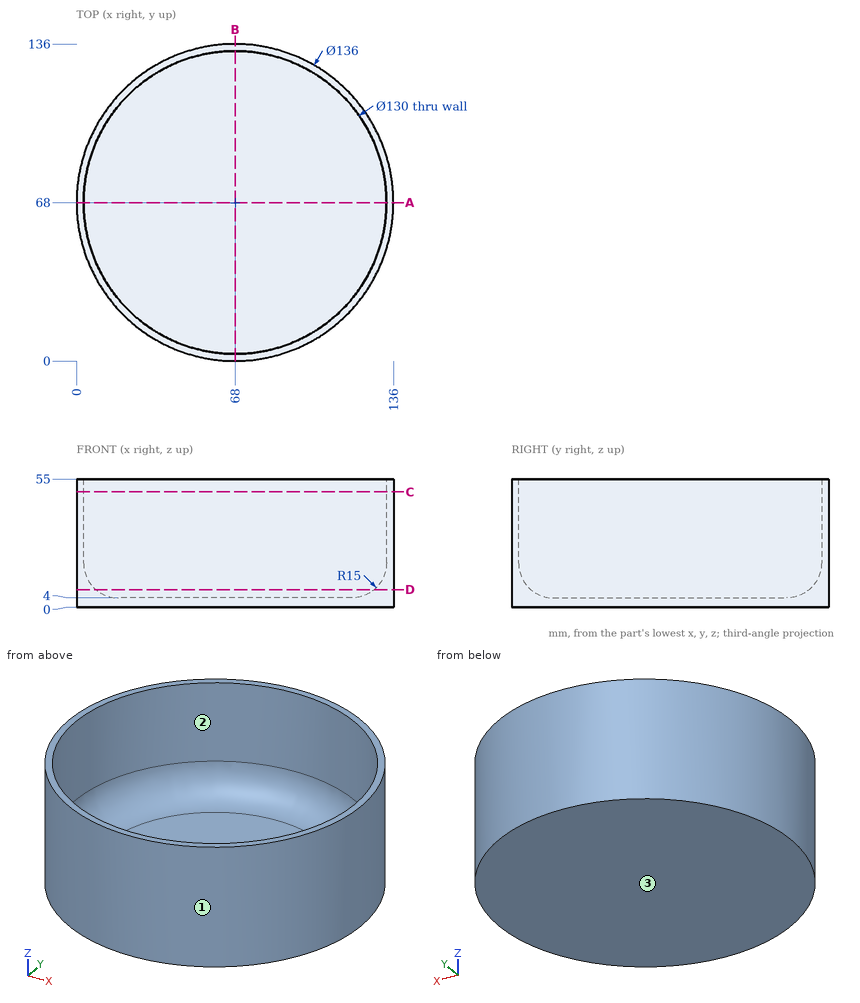
Could you check a few things on this drawing? It's one solid part, dimensions in mm from its lowest x, y, z. Round coordinates to 2 decimals unless told otherwise and drop trailing zeros. Order: outer loops, then holes, each group sorted by start corner. A loop starts at its lowest first (then second) coordinate and runs counter-clockwise, first axis right, second up. Notation, with made-up numbers: M 64,-8.5 L 102,-8.5 A31 cw 102,23.5 Z; hole C 0.25,10.5 d2. An arc over 180 degrees is marked long. Return JSON: item names as keys, results as strings. Group by question number.
1. I'm going to push flat-ended pins straight in: pin 1 Ø1.5 at (x, z) = (61, 36) entering from -Y; pin 2 Ø12 at (x, y) = (81, 30) entering from -Z; pin 3 Ø3 at (x, z) = (108, 48.5) entering from +Y; pin 4 Ø3 at (x, z) = (49.5, 45.5) entering from +Y. Where does each tip first touch, or does it pass through?
2. If we section it at A-A on y = 68: List the corners of the cut face in (x, z) for me, then the cut area to 3 significant figures.
3. If we section it at C-C on z = 49.5: List the corners of the cut face in (x, y) for me.
4. Please list where these lines run through material, in increasing order: probe 1 along Y at (x, z) = (68, 33); probe 2 along Z at (x, y) = (60.5, 104.5); probe 3 along X at (y, z) = (78, 46).
5. If we mould it in two halves opening along Y, with no side actions, what happens to the marked faces 1, 2 and 3? For each: pulls with the +Y half, pulls with the -Y half, needs draft (parallel to the pull), parting line crosses it, or undercut.
6. If we section it at D-D on z = 7.5: List the corners of the cut face in (x, y) for me, then the cut area to 3 significant figures.
Reply:
{
 "1": {"pin 1": "y = 0.29", "pin 2": "z = 0", "pin 3": "y = 124.05", "pin 4": "y = 133.84"},
 "2": {"outline": "M 0,0 L 136,0 L 136,55 L 133,55 L 133,19 A15 cw 118,4 L 18,4 A15 cw 3,19 L 3,55 L 0,55 Z", "area": "947 mm^2"},
 "3": {"outline": "C 68,68 d136; hole C 68,68 d130"},
 "4": {"probe 1": "0 to 3, 133 to 136", "probe 2": "0 to 4", "probe 3": "0.74 to 3.77, 132.23 to 135.26"},
 "5": {"face 1": "parting line crosses it", "face 2": "undercut", "face 3": "needs draft"},
 "6": {"outline": "C 68,68 d136; hole C 68,68 d119.26", "area": "3,360 mm^2"}
}
